The listing builds one solid part. Answer for the finished solid, in the listing's coordinates (mm). A direction names the side the tool comes from. Coordinates: 2 decimals unless noted, no trailing zeros. Order: outer loops, then holes, each group sorted by start corner. A loop starts at its lowest first (then second) coordinate and runs counter-clockwise, first axis right, second up. Notation, with made-up numbers: (75.25, 4) -> (98.25, 4) arc R34 ccw to (98.25, 41) -> close; hole circle Ø2 at (20, 13.25). An arc over 180 degrees is marked (long way). Write each question's results on one line, items separated by ' | '. Start each with the question number.
(1) Given pin 1 (1.5 mm diameter, centred on y = 34.5, z = -3, fed in from +X); pin 2 (1 mm diameter, centred on y = 24.5, z = 4.5, fed in from +X); pin 3 (6 mm diameter, centred on x = 3.5, z = 4, fed in from +Y), each flat-ended and moving along its own axis, determine where each tip first touches the part or whether it passes through.
(2) The part is cut by section A-A, the plane x = 0. Give the vertices of the cut face in (y, z), then the cut area to 3 significant figures.
(3) The part is cut by section C-C, the plane z = -4.25. Give the vertices of the cut face in (x, y).
(4) Straight lines are drawn through the part: L1, parallel to Y at x = -0.25, z = 2.5; L2, parallel to X at y = 107, z = -0.25; L3, parallel to X at y = 79, z = 0.5. For each, find the intervals that lie inside material, in ascending order.
(5) The part is cut by section B-B, the plane y = 33. Give the vertices of the cut face in (x, z).
(6) A tool of negligible diameter and unlimited length cuts with its end or side. For faces 1 (the face through (0, 80, 3)), 2 (the face through (0, 140, 0)), from which of +Z, -Z, +X, -X, +Y, -Y can it reach the whole face along a straight path? Write none if from no direction.
```python
from build123d import *

# Parameters (mm, degrees)
SKETCH1_R   = 0.75
PIN_1_DEPTH = 6
SKETCH2_R   = 0.75
PIN_2_DEPTH = 6
BODY_START  = 6
SKETCH3_R   = 6
BODY_DEPTH  = 74
CABLE_START = 80
SKETCH4_R   = 2
CABLE_DEPTH = 60


with BuildPart() as part:
    # Sketch1 → Pin_1 (new body)
    with BuildSketch(Plane(origin=(0, 0, 0), x_dir=(1, 0, 0), z_dir=(0, 1, 0))):
        with Locations(Location((-2.5, 0, 0), (0, 0, 270))):
            Circle(SKETCH1_R)
    extrude(amount=PIN_1_DEPTH)



with BuildPart() as body_2:
    # Sketch2 → Pin_2 (new body)
    with BuildSketch(Plane(origin=(0, 0, 0), x_dir=(1, 0, 0), z_dir=(0, 1, 0))):
        with Locations(Location((2.5, 0, 0), (0, 0, 270))):
            Circle(SKETCH2_R)
    extrude(amount=PIN_2_DEPTH)


with BuildPart() as part_1:
    add(part.part)

    add(body_2.part)  # Body merges body 2
    # Sketch3 → Body (add)
    with BuildSketch(Plane(origin=(0, 0, 0), x_dir=(1, 0, 0), z_dir=(0, 1, 0)).offset(BODY_START)):
        with Locations(Location((0, 0, 0), (0, 0, 270))):
            Circle(SKETCH3_R)
    extrude(amount=BODY_DEPTH)

    # Sketch4 → Cable (add)
    with BuildSketch(Plane(origin=(0, 0, 0), x_dir=(1, 0, 0), z_dir=(0, 1, 0)).offset(CABLE_START)):
        with Locations(Location((0, 0, 0), (0, 0, 270))):
            Circle(SKETCH4_R)
    extrude(amount=CABLE_DEPTH)


solid = part_1.part
```
Established:
1) pin 1: stops at x = 5.56 | pin 2: stops at x = 4.47 | pin 3: stops at y = 80
2) outline: (6, -6) -> (80, -6) -> (80, -2) -> (140, -2) -> (140, 2) -> (80, 2) -> (80, 6) -> (6, 6) -> close | area: 1,130 mm^2
3) outline: (-4.24, 6) -> (4.24, 6) -> (4.24, 80) -> (-4.24, 80) -> close
4) L1: y = 6 to 80 | L2: x = -1.98 to 1.98 | L3: x = -5.98 to 5.98
5) outline: circle Ø12 at (0, 0)
6) face 1: +Y | face 2: +Z, -Z, +X, -X, +Y
